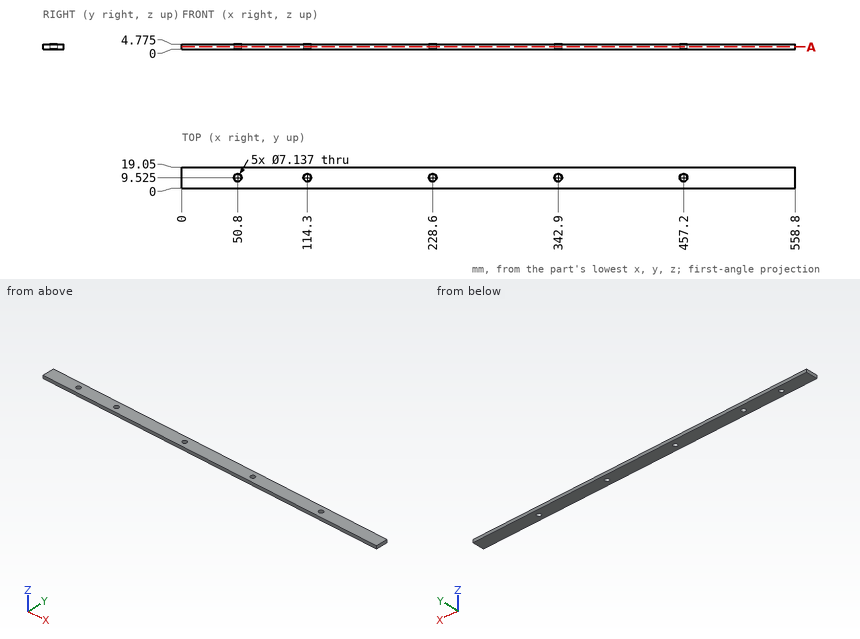
Part print with two shaded views. Sizes in mm from the minimum x, y, z corner. Round coordinates to 2 decimals unless told otherwise and drop trailing zeros. Put each result on its own line as item: value.
Item 1: Slice it at A-A, the plane z = 2.05. Count the separate pieces of the cut face and the enclosed holes in it, plus the area to 3 significant figures.
Here are the results:
separate pieces: 1
enclosed holes: 5
area: 10,400 mm^2
Item 2: Flat gauge pin, fed straight in: P1, Ø6.5, axis at x = 114.3, y = 9.525, coming from the -Z side. Where does the tip first touch, or does it go through?
Here are the results:
P1: passes through
Item 3: Wall check: probe 1 along Y at (x, z) = (342.9, 2.7); probe 2 along X at (y, z) = (7.75, 4.2) (1 decimal); probe 3 along X at (y, z) = (6.75, 2.8) (1 decimal). Give the ranges that are in metal, low to high. Write a range as from..to.
Here are the results:
probe 1: y = 0..5.96, 13.09..19.05
probe 2: x = 0..47.7, 53.9..111.2, 117.4..225.5, 231.7..339.8, 346..454.1, 460.3..558.8
probe 3: x = 0..48.6, 53..112.1, 116.5..226.4, 230.8..340.7, 345.1..455, 459.4..558.8
